Autodesk Inventor part; units mm, degrees
ref_plane "YZ Plane" through (0, 0, 0) normal (1, 0, 0) x (0, 1, 0)
ref_plane "XZ Plane" through (0, 0, 0) normal (0, 1, 0) x (-1, 0, 0)
ref_plane "XY Plane" through (0, 0, 0) normal (0, 0, 1) x (1, 0, 0)
sketch "Szkic1" plane through (0, 0, 0) normal (0, 1, 0) x (-1, 0, 0)
  circle A0 centre (0, 0) radius 14
  dimension "d0" = 28
extrude "Wyciągnięcie proste1" add sketch "Szkic1" along normal blind 2
sketch "Szkic2" plane through (0, 2, 0) normal (0, 1, 0) x (1, 0, 0)
  circle A0 centre (0, 0) radius 12.5
  dimension "d3" = 25
extrude "Wyciągnięcie proste2" add sketch "Szkic2" along normal blind 6
sketch "Szkic3" plane through (0, 8, 0) normal (0, 1, 0) x (1, 0, 0)
  circle A0 centre (1, -6) radius 1.5
  point P0 (0, 0)
  dimension "d6" = 3
  dimension "d10" = 6
  dimension "d11" = 1
extrude "Wyciągnięcie proste3" cut sketch "Szkic3" against normal up to surface (8 mm away)
mirror "Odbij1" about plane through (0, 0, 0) normal (0, 0, 1) of "Wyciągnięcie proste3"
sketch "Sketch5" plane through (0, 8, 0) normal (0, 1, 0) x (1, 0, 0)
  arc A0 (3.12, 1.59) -> (3.12, -1.59) centre (1, 0) ccw
  line L0 (3.12, -1.59) -> (3.12, 1.59)
  point P0 (0, 0)
  dimension "d12" = 5.3
  dimension "d13" = 3.18
  dimension "d14" = 1
  dimension "d15" = 0
extrude "Extrusion4" cut sketch "Sketch5" against normal up to surface (8 mm away)
properties part number "InputShaft2_3DPrint"
Can you work these out from the model? Positions are in its coordinate system, mm. Coordinates: 2 decimals unless noted, no trailing zeros. Order: outer loops, then holes, each group sorted by start corner. A loop starts at its lowest first (then second) coordinate and runs counter-clockwise, first axis right, second up. Notation, with made-up numbers: (47, 74) - (96, 74) arc R25 cw to (96, 105) - close; hole circle Ø2 at (15, 60). An arc over 180 degrees is marked (long way). Answer as a JSON object with one key per item and string values. Group by question number.
Q1. Will these pins go through, and if not, where does the flat tip stop? P1, Ø1.5, axis at x = -7, y = 5, coming from the -Z side; P2, Ø2.5, axis at y = 4.5, z = -0.5, coming from the -X side; P3, Ø1.5, axis at x = -4, y = 3.5, coming from the -Z side.
Q2. Imagine slicing it at D-D (x = 10.5). Please give me the cut outline in (y, z), and give its area (3 significant figures).
Q3. Imagine slicing it at A-A (y = 1.5). Please give me the cut outline in (x, z).
Q4. Imagine slicing it at B-B (x = -1). Please give me the cut outline in (y, z).
Q5. We'd pull the mould along Z, two halves only. Please class faces 1 (the face through (5.3, 2, 11.5)), 2 (the face through (11.923, 4.958, 3.755)), 3 (the face through (3.12, 4, 0)), 4 (the face through (2.386, 4.056, -5.425)): +Z half, -Z half, draft (parallel to the pull), parting line (faces both ways), or undercut.
Q6. I need wall thicknesses on line 1 (X direction, y = 4.5, z = 0); line 2 (Z direction, x = 1, y = 5.75); line 3 (Y direction, x = 12.5, z = 5.5). Which ranges of each line are inside material? Lowest first, please. Write a range as from..to.
Q7. Imagine slicing it at C-C (z = -6). Please give me the cut outline in (x, y).
Determined:
{
 "1": {"P1": "stops at z = -10.83", "P2": "stops at x = -12.5", "P3": "stops at z = -12.07"},
 "2": {"outline": "(0, -9.26) - (2, -9.26) - (2, -6.78) - (8, -6.78) - (8, 6.78) - (2, 6.78) - (2, 9.26) - (0, 9.26) - close", "area": "118 mm2"},
 "3": {"outline": "circle Ø28 at (0, 0); hole circle Ø3 at (1, -6); hole circle Ø3 at (1, 6); hole (3.12, -1.59) - (3.12, 1.59) arc R2.65 ccw (long way) to start"},
 "4": {"outline": "(0, -13.96) - (2, -13.96) - (2, -12.46) - (8, -12.46) - (8, -1.74) - (0, -1.74) - close; (0, 1.74) - (8, 1.74) - (8, 12.46) - (2, 12.46) - (2, 13.96) - (0, 13.96) - close"},
 "5": {"face 1": "draft", "face 2": "parting line", "face 3": "undercut", "face 4": "undercut"},
 "6": {"line 1": "x = -12.5..-1.65, 3.12..12.5", "line 2": "z = -12.46..-7.5, -4.5..-2.65, 2.65..4.5, 7.5..12.46", "line 3": "y = 0..2"},
 "7": {"outline": "(-12.65, 0) - (-0.5, 0) - (-0.5, 8) - (-10.97, 8) - (-10.97, 2) - (-12.65, 2) - close; (2.5, 0) - (12.65, 0) - (12.65, 2) - (10.97, 2) - (10.97, 8) - (2.5, 8) - close"}
}
